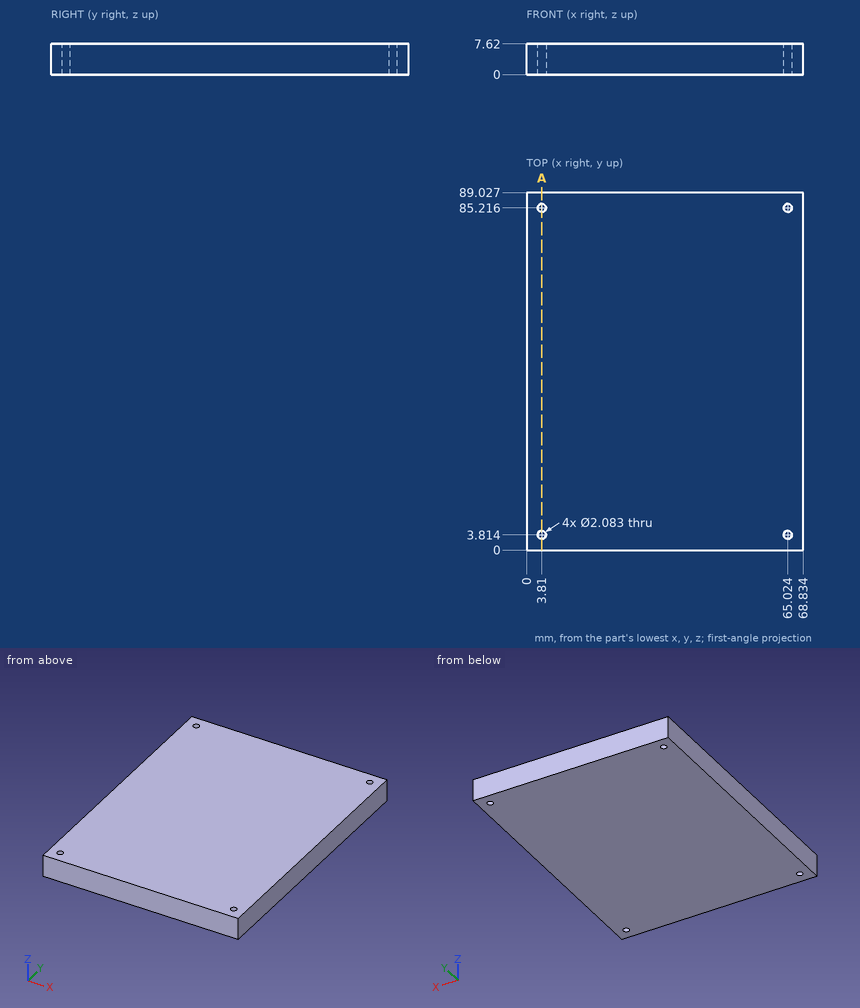
Can you work these out from the drawing? Everything is in mm from the part's minimum corner. Round coordinates to 2 decimals unless told otherwise and drop trailing zeros. Write each loop counter-clockwise with the first axis right and the second up, starting at its lowest first coordinate (ties: lowest second). Pieces come first, ordered by that corner, then holes. Notation, with made-up numbers: (-18.5, 22.25) - (-4.5, 22.25) arc R14 cw to (-4.5, 32.25) - close; hole circle Ø9 at (-6.75, 52). An arc over 180 degrees is marked (long way). Put each result on its own line as item: value. Start each with the question number.
(1) I want a section at A-A, the plane x = 3.81. Please give me the cut outline in (y, z) (1 decimal).
(2) Will these pins go through, and if not, where does the flat tip stop? pin 1 (6 mm diameter, centred on x = 47.5, y = 16, fed in from -Z); pin 2 (1.7 mm diameter, centred on x = 65.024, y = 85.216, fed in from +Z).
(3) I need wall thicknesses on probe 1 along Y at (x, z) = (3.81, 3.75) (1 decimal); probe 2 along Y at (x, z) = (3.5, 6.5). Which ranges of each line are inside material? Lowest first, please.
Here are the results:
1. outline: (0, 0) - (2.8, 0) - (2.8, 7.6) - (0, 7.6) - close; (4.9, 0) - (84.2, 0) - (84.2, 7.6) - (4.9, 7.6) - close; (86.3, 0) - (89, 0) - (89, 7.6) - (86.3, 7.6) - close
2. pin 1: stops at z = 0
2. pin 2: passes through
3. probe 1: y = 0 to 2.8, 4.9 to 84.2, 86.3 to 89
3. probe 2: y = 0 to 2.82, 4.81 to 84.22, 86.21 to 89.03
